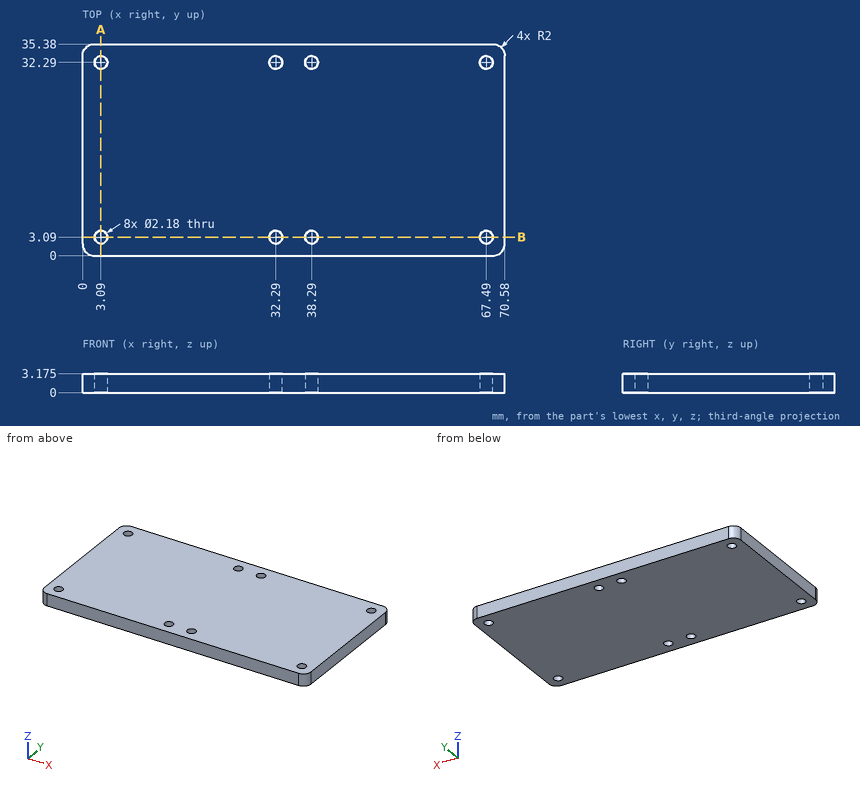
Check sheet for the drawn part. Datum: minimum x, y, z corner. Units: mm. Coordinates: 2 decimals unless noted, no trailing zeros. Write each loop counter-clockwise with the first axis right and the second up, starting at its lowest first coordinate (ties: lowest second). Pieces come first, ordered by that corner, then holes. Notation, with made-up numbers: M 81.25,-33.75 L 105.25,-33.75 A28 cw 105.25,-13.75 Z; hole C -3.5,29.5 d4. An arc over 180 degrees is marked long. Use a Markdown table: item, result.
Q1. Sectioned sample at A-A, the plane x = 3.09. Record the boundary of the cut face in (y, z) (3 decimals), plus the area to 3 significant figures.
Reply:
| item | result |
|---|---|
| outline | M 0,0 L 2,0 L 2,3.175 L 0,3.175 Z; M 4.18,0 L 31.2,0 L 31.2,3.175 L 4.18,3.175 Z; M 33.38,0 L 35.38,0 L 35.38,3.175 L 33.38,3.175 Z |
| area | 98.5 mm² |
Q2. Thickness scan on line 1 (X direction, y = 32.29, z = 1.9); line 2 (Y direction, x = 38.29, z = 1.85); line 3 (X direction, y = 32, z = 0.5). Record the ranges inside material, lowest first.
Reply:
| item | result |
|---|---|
| line 1 | x = 0 to 2, 4.18 to 31.2, 33.38 to 37.2, 39.38 to 66.4, 68.58 to 70.58 |
| line 2 | y = 0 to 2, 4.18 to 31.2, 33.38 to 35.38 |
| line 3 | x = 0 to 2.04, 4.14 to 31.24, 33.34 to 37.24, 39.34 to 66.44, 68.54 to 70.58 |
Q3. Sectioned sample at B-B, the plane y = 3.09. Record the boundary of the cut face in (x, z) (3 decimals), plus the area to 3 significant figures.
Reply:
| item | result |
|---|---|
| outline | M 0,0 L 2,0 L 2,3.175 L 0,3.175 Z; M 4.18,0 L 31.2,0 L 31.2,3.175 L 4.18,3.175 Z; M 33.38,0 L 37.2,0 L 37.2,3.175 L 33.38,3.175 Z; M 39.38,0 L 66.4,0 L 66.4,3.175 L 39.38,3.175 Z; M 68.58,0 L 70.58,0 L 70.58,3.175 L 68.58,3.175 Z |
| area | 196 mm² |
